Check sheet for the modelled part. Datum: model origin and axes. Units: mm. Face numbers are marked on the shaded views. Round coordinates to 2 decimals unless told otherwise and drop trailing zeros. Write each loop counter-clockwise with the first axis right and the second up, starting at its lowest first coordinate (ties: lowest second). Pieces come first, ordered by that corner, then holes. Notation, with made-up numbers: (12, 73.5) - (64, 73.5) arc R28 cw to (64, 100.5) - close; hole circle Ø2 at (34, 29). An arc over 180 degrees is marked (long way). Use one line per item in the form item = value. Start each with the question number.
1) Section check B-B (y = 0). Record the boundary of the cut face in (x, z).
2) Gauge pin test, flat ends, axial feed: P1, Ø0.6, axis at x = -18.5, z = 130, coming from the -Y side; P2, Ø3, axis at x = -1, y = -25.5, coming from the -Z side; P3, Ø1, axis at y = 18.5, z = 127, coming from the +X side. Record the tip position at first contact, or that the pin passes through.
3) Draft check along Z on the marked faces 1, 2 and 3. Enter one of: +Z half, -Z half, draft (parallel to the pull), parting line (faces both ways), or undercut.
4) Scan lines: probe 1 along Y at (x, z) = (16, 164.5); probe 2 along Z at (x, y) = (11, -20); probe 3 along X at (y, z) = (1, 87.5). Record each from-to range of solid material in increasing order.
from build123d import *
from build123d.topology import SkipClean

# Parameters (mm, degrees)
SKETCH1_R           = 22.5
BOSS_EXTRUDE1_DEPTH = 200
BOSS_EXTRUDE2_START = 50
BOSS_EXTRUDE2_DEPTH = 100
BOSS_EXTRUDE3_START = -50
SKETCH4_R           = 23.75
SKETCH4_R_2         = 22.5
BOSS_EXTRUDE3_DEPTH = 5
BOSS_EXTRUDE4_START = -155
SKETCH4_2_R         = 23.75
SKETCH4_2_R_2       = 22.5
BOSS_EXTRUDE4_DEPTH = 5


with BuildPart() as part:
    # Sketch1 → Boss-Extrude1 (new body)
    with BuildSketch(Plane.XY):
        Circle(SKETCH1_R)
        with BuildLine():
            Line((-3.5, 19.691368668), (-3.5, 17.656443583))
            ThreePointArc((-3.5, 17.656443583), (-6.888301783, 16.629831585), (-10.010117255, 14.959864723))
            Line((-10.010117255, 14.959864723), (-11.449026581, 16.39877405))
            ThreePointArc((-11.449026581, 16.39877405), (-14.142135624, 14.142135624), (-16.39877405, 11.449026581))
            Line((-16.39877405, 11.449026581), (-14.959864723, 10.010117255))
            ThreePointArc((-14.959864723, 10.010117255), (-16.629831585, 6.888301783), (-17.656443583, 3.5))
            Line((-17.656443583, 3.5), (-19.691368668, 3.5))
            ThreePointArc((-19.691368668, 3.5), (-20, 0), (-19.691368668, -3.5))
            Line((-19.691368668, -3.5), (-17.656443583, -3.5))
            ThreePointArc((-17.656443583, -3.5), (-16.629831585, -6.888301783), (-14.959864723, -10.010117255))
            Line((-14.959864723, -10.010117255), (-16.39877405, -11.449026581))
            ThreePointArc((-16.39877405, -11.449026581), (-14.142135624, -14.142135624), (-11.449026581, -16.39877405))
            Line((-11.449026581, -16.39877405), (-10.010117255, -14.959864723))
            ThreePointArc((-10.010117255, -14.959864723), (-6.888301783, -16.629831585), (-3.5, -17.656443583))
            Line((-3.5, -17.656443583), (-3.5, -19.691368668))
            ThreePointArc((-3.5, -19.691368668), (0, -20), (3.5, -19.691368668))
            Line((3.5, -19.691368668), (3.5, -17.656443583))
            ThreePointArc((3.5, -17.656443583), (6.888301783, -16.629831585), (10.010117255, -14.959864723))
            Line((10.010117255, -14.959864723), (11.449026581, -16.39877405))
            ThreePointArc((11.449026581, -16.39877405), (14.142135624, -14.142135624), (16.39877405, -11.449026581))
            Line((16.39877405, -11.449026581), (14.959864723, -10.010117255))
            ThreePointArc((14.959864723, -10.010117255), (16.629831585, -6.888301783), (17.656443583, -3.5))
            Line((17.656443583, -3.5), (19.691368668, -3.5))
            ThreePointArc((19.691368668, -3.5), (20, 0), (19.691368668, 3.5))
            Line((19.691368668, 3.5), (17.656443583, 3.5))
            ThreePointArc((17.656443583, 3.5), (16.629831585, 6.888301783), (14.959864723, 10.010117255))
            Line((14.959864723, 10.010117255), (16.39877405, 11.449026581))
            ThreePointArc((16.39877405, 11.449026581), (14.142135624, 14.142135624), (11.449026581, 16.39877405))
            Line((11.449026581, 16.39877405), (10.010117255, 14.959864723))
            ThreePointArc((10.010117255, 14.959864723), (6.888301783, 16.629831585), (3.5, 17.656443583))
            Line((3.5, 17.656443583), (3.5, 19.691368668))
            ThreePointArc((3.5, 19.691368668), (0, 20), (-3.5, 19.691368668))
        make_face(mode=Mode.SUBTRACT)
    extrude(amount=BOSS_EXTRUDE1_DEPTH)

    # Sketch3 → Boss-Extrude2 (add)
    with BuildSketch(Plane.XY.offset(BOSS_EXTRUDE2_START)):
        with BuildLine():
            Line((-2, 23.665639649), (-0.800587161, 26.237788783))
            ThreePointArc((-0.800587161, 26.237788783), (0, 26.25), (0.800587161, 26.237788783))
            Line((0.800587161, 26.237788783), (2, 23.665639649))
            ThreePointArc((2, 23.665639649), (2.751390898, 23.590090041), (3.5, 23.490689645))
            Line((3.5, 23.490689645), (3.5, 22.226110771))
            ThreePointArc((3.5, 22.226110771), (0, 22.5), (-3.5, 22.226110771))
            Line((-3.5, 22.226110771), (-3.5, 23.490689645))
            ThreePointArc((-3.5, 23.490689645), (-2.751390898, 23.590090041), (-2, 23.665639649))
        make_face()
        with BuildLine():
            Line((17.498376555, 14.144144299), (18.593533985, 14.776433736))
            ThreePointArc((18.593533985, 14.776433736), (19.053921804, 14.177819434), (19.495045133, 13.564870632))
            Line((19.495045133, 13.564870632), (22.322298044, 13.812223211))
            ThreePointArc((22.322298044, 13.812223211), (22.733166849, 13.125), (23.122885205, 12.425565572))
            Line((23.122885205, 12.425565572), (21.495045133, 10.100769017))
            ThreePointArc((21.495045133, 10.100769017), (21.805312702, 9.412270607), (22.093533985, 8.714255909))
            Line((22.093533985, 8.714255909), (20.998376555, 8.081966472))
            ThreePointArc((20.998376555, 8.081966472), (19.485571585, 11.25), (17.498376555, 14.144144299))
        make_face()
        with BuildLine():
            Line((20.998376555, -8.081966472), (22.093533985, -8.714255909))
            ThreePointArc((22.093533985, -8.714255909), (21.805312702, -9.412270607), (21.495045133, -10.100769017))
            Line((21.495045133, -10.100769017), (23.122885205, -12.425565572))
            ThreePointArc((23.122885205, -12.425565572), (22.733166849, -13.125), (22.322298044, -13.812223211))
            Line((22.322298044, -13.812223211), (19.495045133, -13.564870632))
            ThreePointArc((19.495045133, -13.564870632), (19.053921804, -14.177819434), (18.593533985, -14.776433736))
            Line((18.593533985, -14.776433736), (17.498376555, -14.144144299))
            ThreePointArc((17.498376555, -14.144144299), (19.485571585, -11.25), (20.998376555, -8.081966472))
        make_face()
        with BuildLine():
            Line((3.5, -22.226110771), (3.5, -23.490689645))
            ThreePointArc((3.5, -23.490689645), (2.751390898, -23.590090041), (2, -23.665639649))
            Line((2, -23.665639649), (0.800587161, -26.237788783))
            ThreePointArc((0.800587161, -26.237788783), (0, -26.25), (-0.800587161, -26.237788783))
            Line((-0.800587161, -26.237788783), (-2, -23.665639649))
            ThreePointArc((-2, -23.665639649), (-2.751390898, -23.590090041), (-3.5, -23.490689645))
            Line((-3.5, -23.490689645), (-3.5, -22.226110771))
            ThreePointArc((-3.5, -22.226110771), (0, -22.5), (3.5, -22.226110771))
        make_face()
        with BuildLine():
            Line((-17.498376555, -14.144144299), (-18.593533985, -14.776433736))
            ThreePointArc((-18.593533985, -14.776433736), (-19.053921804, -14.177819434), (-19.495045133, -13.564870632))
            Line((-19.495045133, -13.564870632), (-22.322298044, -13.812223211))
            ThreePointArc((-22.322298044, -13.812223211), (-22.733166849, -13.125), (-23.122885205, -12.425565572))
            Line((-23.122885205, -12.425565572), (-21.495045133, -10.100769017))
            ThreePointArc((-21.495045133, -10.100769017), (-21.805312702, -9.412270607), (-22.093533985, -8.714255909))
            Line((-22.093533985, -8.714255909), (-20.998376555, -8.081966472))
            ThreePointArc((-20.998376555, -8.081966472), (-19.485571585, -11.25), (-17.498376555, -14.144144299))
        make_face()
        with BuildLine():
            Line((-20.998376555, 8.081966472), (-22.093533985, 8.714255909))
            ThreePointArc((-22.093533985, 8.714255909), (-21.805312702, 9.412270607), (-21.495045133, 10.100769017))
            Line((-21.495045133, 10.100769017), (-23.122885205, 12.425565572))
            ThreePointArc((-23.122885205, 12.425565572), (-22.733166849, 13.125), (-22.322298044, 13.812223211))
            Line((-22.322298044, 13.812223211), (-19.495045133, 13.564870632))
            ThreePointArc((-19.495045133, 13.564870632), (-19.053921804, 14.177819434), (-18.593533985, 14.776433736))
            Line((-18.593533985, 14.776433736), (-17.498376555, 14.144144299))
            ThreePointArc((-17.498376555, 14.144144299), (-19.485571585, 11.25), (-20.998376555, 8.081966472))
        make_face()
    extrude(amount=BOSS_EXTRUDE2_DEPTH)

    # Sketch4 → Boss-Extrude3 (add)
    with SkipClean():  # the faces are left unmerged after this step: merging them gives an invalid solid
        with BuildSketch(Plane.XY.offset(200).offset(BOSS_EXTRUDE3_START)):
            with Locations(Location((0, 0, 0), (0, 0, 180))):
                Circle(SKETCH4_R)
            with Locations(Location((0, 0, 0), (0, 0, 180))):
                Circle(SKETCH4_R_2, mode=Mode.SUBTRACT)
        extrude(amount=BOSS_EXTRUDE3_DEPTH)

    # Sketch4<2> → Boss-Extrude4 (add)
    with SkipClean():  # the faces are left unmerged after this step: merging them gives an invalid solid
        with BuildSketch(Plane.XY.offset(200).offset(BOSS_EXTRUDE4_START)):
            with Locations(Location((0, 0, 0), (0, 0, 180))):
                Circle(SKETCH4_2_R)
            with Locations(Location((0, 0, 0), (0, 0, 180))):
                Circle(SKETCH4_2_R_2, mode=Mode.SUBTRACT)
        extrude(amount=BOSS_EXTRUDE4_DEPTH)


solid = part.part
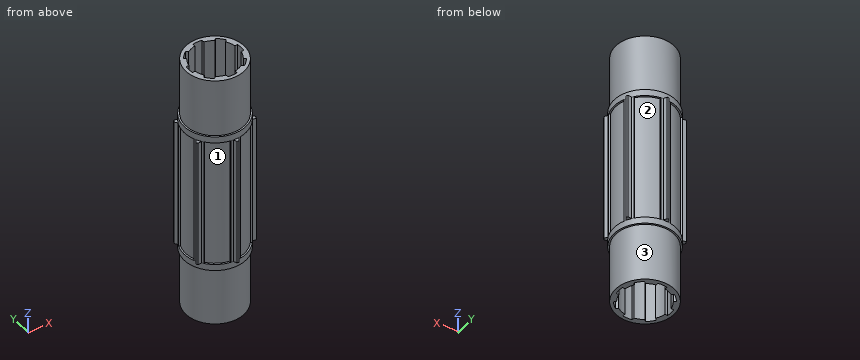
Results are:
q1.outline = (-23.75, 45) - (-22.5, 45) - (-22.5, 0) - (-20, 0) - (-20, 200) - (-22.5, 200) - (-22.5, 155) - (-23.75, 155) - (-23.75, 150) - (-22.5, 150) - (-22.5, 50) - (-23.75, 50) - close; (20, 0) - (22.5, 0) - (22.5, 45) - (23.75, 45) - (23.75, 50) - (22.5, 50) - (22.5, 150) - (23.75, 150) - (23.75, 155) - (22.5, 155) - (22.5, 200) - (20, 200) - close
q2.P1 = -14.78
q2.P2 = 50
q2.P3 = 13.5
q3.face_1 = undercut
q3.face_2 = undercut
q3.face_3 = draft
q4.probe_1 = -15.82 to -12, -11.05 to -8.25, 8.25 to 11.05, 12 to 15.82
q4.probe_2 = 45 to 50, 150 to 155
q4.probe_3 = -22.48 to -19.97, 19.97 to 22.48
